Build history of the part. All positions in model axes, mm. A direction names the side the tool comes from. Give positions to 0.01 mm unless a question says otherwise; leave off trailing zeros. Write each loop counter-clockwise with the first axis right and the second up, starting at its lowest first coordinate (ties: lowest second). Pieces come first, ordered by that corner, then holes. Notation, with made-up numbers: M 8.25,69.25 L 50.25,69.25 A22 cw 50.25,94.25 Z; hole C 31.5,-8.5 d3. An arc over 180 degrees is marked long. One line per item, written item: value. Start each with the question number.
from build123d import *

# Parameters (mm, degrees)
EXTRUDE001_DEPTH      = 4
BOX001_W              = 46
BOX001_H              = 17
BOX001_DEPTH          = 10
SKETCH001_W           = 18.2
SKETCH001_H           = 25.7
EXTRUDE_DEPTH         = 10
EXTRUDE002_DEPTH      = 1
EXTRUDE002_DEPTH_BACK = 1.55


with BuildPart() as bottomboard:
    # Sketch002 → Extrude001 (new body)
    with BuildSketch(Plane.XY):
        Polygon((-0.1, 27.15), (34.579, 27.15), (34.579, 6.313), (25.753, 6.313), (25.753, -0.1), (9.361, -0.1), (9.361, 6.313), (-0.1, 6.313), align=None)
    extrude(amount=-EXTRUDE001_DEPTH)


with BuildPart() as obj1:
    # Box001 → Box001 (new body)
    with BuildSketch(Plane(origin=(-6, 9, -5), x_dir=(1, 0, 0), z_dir=(0, 0, 1))):
        with Locations((23, 8.5)):
            Rectangle(BOX001_W, BOX001_H)
    extrude(amount=BOX001_DEPTH)


with BuildPart() as cutouts:
    # Sketch001 → Extrude (new body, symmetric)
    with BuildSketch(Plane.XY):
        with Locations((17.308148, 19.873965)):
            Rectangle(SKETCH001_W, SKETCH001_H)
    extrude(amount=EXTRUDE_DEPTH, both=True)

    # Fusion: union bottomBoard, obj1
    add(bottomboard.part)
    add(obj1.part)


with BuildPart() as obj2:
    # Sketch003 → Extrude002 (new body, two sides)
    with BuildSketch(Plane.XY) as extrude002_sk:
        with BuildLine():
            ThreePointArc((-1, 37.623965), (-8.071068, 34.695033), (-11, 27.623965))
            Line((-11, 5), (-11, 27.623965))
            ThreePointArc((-11, 5), (-8.071068, -2.071068), (-1, -5))
            Line((35.479, -5), (-1, -5))
            ThreePointArc((35.479, -5), (42.550068, -2.071068), (45.479, 5))
            Line((45.479, 27.623965), (45.479, 5))
            ThreePointArc((45.479, 27.623965), (42.550068, 34.695033), (35.479, 37.623965))
            Line((-1, 37.623965), (35.479, 37.623965))
        make_face()
    extrude(amount=EXTRUDE002_DEPTH)
    extrude(extrude002_sk.sketch, amount=-EXTRUDE002_DEPTH_BACK)

    # Cut: cut CutOuts
    add(cutouts.part, mode=Mode.SUBTRACT)


solid = obj2.part
1) Drop flat-ended pins along their axis: P1, Ø1, axis at y = 30, z = -1, coming from the +X side; P2, Ø1.2, axis at y = 3.5, z = -0.5, coming from the +X side; P3, Ø0.6, axis at x = 31.5, y = 26.5, coming from the -Z side; P4, Ø6, axis at x = 25, y = 28.5, coming from the +Z side. Give the stop position or say it passes through.
2) Mould opens along Y. For faces 4 (the face through (29, 2, -1.55)), 5 (the face through (17, -5, 0)), 6 (the face through (25.753, 3, -1)) say: released by +Y, released by -Y, zero draft, split by the parting line, or undercut.
3) Probe line 1 along X through (y, z) = (16, -0.55); line 2 along Y through (x, z) = (17, -0.1); line 3 along Y through (x, z) = (36, 0.2). List the from-to ranges inside material, lowest first. Write a range as from..to.
4) Band-saw the part on B-B (y = 8). List the corners of the cut face in (x, z).
5) Tool access for faces 1 (the face through (26.408, 29, 0)), 2 (the face through (34.579, 8, -1)), 3 (the face through (42.627, 34.617, -0.257)): list every direction of +Z, -Z, +X, -X, +Y, -Y with a clear straight run to the whole face (end or side of a thin tool).
6) Band-saw the part on C-C (z = -0.6). List the corners of the cut face in (x, y), then the cut area to 3 significant figures.
7) Band-saw the part on D-D (y = 22). List the corners of the cut face in (x, z).
8) Band-saw the part on A-A (x = 27). List the corners of the cut face in (y, z).
Model answer:
1. P1: stops at x = 45.3
1. P2: stops at x = 45.44
1. P3: stops at z = 0
1. P4: stops at z = 1
2. face 4: zero draft
2. face 5: released by -Y
2. face 6: undercut
3. line 1: x = -11..-6, 40..45.48
3. line 2: y = -5..-0.1, 32.72..37.62
3. line 3: y = -4.99..9, 26..37.61
4. outline: M -11,-1.55 L -0.1,-1.55 L -0.1,0 L 8.21,0 L 8.21,1 L -11,1 Z; M 26.41,0 L 34.58,0 L 34.58,-1.55 L 45.48,-1.55 L 45.48,1 L 26.41,1 Z
5. face 1: +Z, -Z
5. face 2: -Z
5. face 3: +Z, -Z, +X, +Y
6. outline: M -11,5 A10 ccw -1,-5 L 35.48,-5 A10 ccw 45.48,5 L 45.48,27.62 A10 ccw 35.48,37.62 L -1,37.62 A10 ccw -11,27.62 Z; hole M -6,9 L -0.1,9 L -0.1,6.31 L 9.36,6.31 L 9.36,-0.1 L 25.75,-0.1 L 25.75,6.31 L 34.58,6.31 L 34.58,9 L 40,9 L 40,26 L 34.58,26 L 34.58,27.15 L 26.41,27.15 L 26.41,32.72 L 8.21,32.72 L 8.21,27.15 L -0.1,27.15 L -0.1,26 L -6,26 Z
6. area: 1,200 mm²
7. outline: M -11,-1.55 L -6,-1.55 L -6,1 L -11,1 Z; M 40,-1.55 L 45.48,-1.55 L 45.48,1 L 40,1 Z
8. outline: M -5,-1.55 L 6.31,-1.55 L 6.31,0 L 9,0 L 9,1 L -5,1 Z; M 26,0 L 27.15,0 L 27.15,-1.55 L 37.62,-1.55 L 37.62,1 L 26,1 Z
